Build history of the part. All positions in model axes, mm. Face numbers are marked on the shaded views. A direction names the side the tool comes from. Round coordinates to 2 decimals unless told otherwise and drop trailing zeros. Write each loop counter-clockwise with the first axis right and the second up, starting at its lowest first coordinate (ties: lowest second). Pieces come first, ordered by that corner, then holes.
Autodesk Fusion 360 part; units mm, degrees
sketch "Sketch1" plane through (0, 0, 0) normal (0, 0, 1) x (1, 0, 0)
  line L0 (60, -7.5) -> (-60, -7.5)
  line L1 (-60, -7.5) -> (-60, 7.5)
  line L2 (-60, 7.5) -> (60, 7.5)
  line L3 (60, 7.5) -> (60, -7.5)
  line L4 (60, 7.5) -> (60, 57.5)
  circle A0 centre (30, 57.5) radius 30
  circle A1 centre (30, 57.5) radius 20
  line L5 (10.9888, 80.7072) -> (-60, 7.5)
  dimension "d1" = 120
  dimension "d2" = 15
  dimension "d5" = 30
  dimension "d6" = 60
  dimension "d7" = 40
extrude "Extrude1" add sketch "Sketch1" along normal blind 40 contours A0 L5 picked at (10.8489, 75.8663)
extrude "Extrude2" add sketch "Sketch1" along normal blind 20 contours L2 L4 A0 L5
extrude "Extrude3" add sketch "Sketch1" along normal blind 60 contours L0 L1 L2 L3
sketch "Sketch2" plane through (-60, 0, 0) normal (-1, 0, 0) x (0, -1, 0)
  line L0 (-7.5, 0) -> (7.5, 0)
  line L1 (7.5, 0) -> (7.5, 60)
  line L2 (7.5, 60) -> (-7.5, 60)
  line L3 (-7.5, 60) -> (-7.5, 20)
  line L4 (-7.5, 20) -> (-7.5, 0)
  line L5 (7.5, 19.588) -> (0, 19.588)
  line L6 (0, 19.588) -> (0, 45)
  line L7 (0, 45) -> (7.5, 45)
  line L8 (7.5, 45) -> (7.5, 19.588)
extrude "Extrude4" cut sketch "Sketch2" against normal blind 120 contours L1 L5 L6 L7 L8
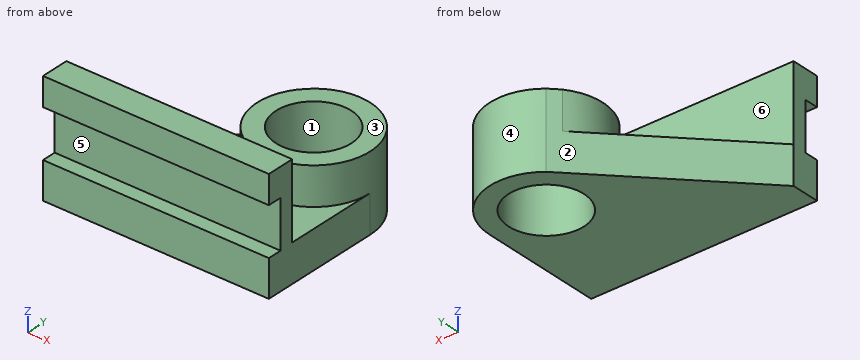
1) Slice it at A-A (x = 30). Write the cut outline in (y, z).
Results:
outline: (-7.5, 0) - (37.5, 0) - (37.5, 40) - (27.5, 40) - (27.5, 20) - (7.5, 20) - (7.5, 60) - (-7.5, 60) - (-7.5, 45) - (0, 45) - (0, 19.59) - (-7.5, 19.59) - close; (77.5, 0) - (87.5, 0) - (87.5, 40) - (77.5, 40) - close
2) Mould opens along X. For the marked faces 1, 2 and 3 say: released by +X, released by -X, zero draft, split by the parting line, or undercut.
Results:
face 1: undercut
face 2: released by -X
face 3: zero draft
3) Which spindle directions (+Z, -Z, +X, -X, +Y, -Y) get a long thin tool onto all of the face, cutting with end or side? Do the marked faces 4, 5 and 6. Say none if no direction does.
Results:
face 4: +Z
face 5: +X, -X, -Y
face 6: +Z, +X, -X
4) Wall check: L1, parallel to Y at x = 30, z = 11; L2, parallel to X at y = 57, z = 32; L3, parallel to Y at x = 38, z = 33.5. Give the ranges that are in metal, low to high.
Results:
L1: y = -7.5 to 37.5, 77.5 to 87.5
L2: x = 0 to 10.01, 49.99 to 60
L3: y = 0 to 7.5, 28.59 to 39.17, 75.83 to 86.41
5) Slice it at B-B (z = 7.5). Write the cut outline in (x, y).
Results:
outline: (-60, -7.5) - (60, -7.5) - (60, 57.5) arc R30 ccw to (10.99, 80.71) - (-60, 7.5) - close; hole circle Ø40 at (30, 57.5)
6) Pin check, flat tips, straight feed: pin 1 Ø6 at (x, z) = (46.5, 32) entering from +Y; pin 2 Ø3 at (x, z) = (19, 37.5) entering from -Y; pin 3 Ø18 at (x, y) = (26, 52) entering from +Z; pin 4 Ø20.5 at (x, y) = (-6.5, 51.5) entering from +Z. Stop position of each tip, or through.
Results:
pin 1: stops at y = 84.29
pin 2: stops at y = 0
pin 3: passes through
pin 4: stops at z = 40
7) Slice it at C-C (y = 68). Write the cut outline in (x, z).
Results:
outline: (-1.33, 0) - (12.98, 0) - (12.98, 40) - (1.9, 40) - (1.9, 20) - (-1.33, 20) - close; (47.02, 0) - (58.1, 0) - (58.1, 40) - (47.02, 40) - close
8) Slice it at D-D (z = 23). Write the cut outline in (x, y).
Results:
outline: (-60, 0) - (60, 0) - (60, 7.5) - (-60, 7.5) - close; (6.22, 75.79) arc R30 ccw (long way) to (10.99, 80.71) - close; hole circle Ø40 at (30, 57.5)
